Work out the finished part from the listing and answer in its coordinate system (mm). Face numbers are marked on the shaded views. A direction names the side the tool comes from. Give positions to 0.01 mm unless a question says otherwise; leave off trailing zeros. Loops run counter-clockwise (first coordinate to the right, second up) from the corner with the lowest first, then second, coordinate; pieces in that order, holes last. Notation, with made-up numbers: (49.5, 5.5) - (66.5, 5.5) arc R24 cw to (66.5, 28.5) - close; hole circle Ø5 at (-19, -13.75). An arc over 180 degrees is marked (long way). One line per question, with ' | ' between items. Start each with the question number.
1. Which of the six approach directions +Z, -Z, +X, -X, +Y, -Y give full straight-line access (tool end or side, diameter ignored) to the marked faces 1, 2 and 3?
2. Section A-A (y = 28) is taken. Determine the outline of the cut face in (x, z), plus the area to 3 significant figures.
3. Section C-C (y = 83.5) is taken. Determine the outline of the cut face in (x, z), plus the area to 3 significant figures.
4. Each of these flat-tipped pins is pushed along its axis until it touches: pin 1 (0.8 mm diameter, centred on y = 124.5, z = 1.5, fed in from -X); pin 2 (2 mm diameter, centred on y = 72.5, z = 1.5, fed in from +X); pin 3 (8 mm diameter, centred on x = 30, y = 124, fed in from -Z). Where does it stop, or does it pass through?
5. Section D-D (x = -2) is taken. Determine the outline of the cut face in (y, z).
6. Section B-B (x = 10) is taken. Determine the outline of the cut face in (y, z).
7. Find the intervals of material crossed by line 1 (Y direction, x = 10, z = 1); line 2 (X direction, y = 28, z = 0.75); line 3 (X direction, y = 42, z = 1.5), in increasing order.
from build123d import *

# Parameters (mm, degrees)
F1_DEPTH       = 3.5
F3_DEPTH       = 2.5
F5_D           = 4.5
F5_CSINK_D     = 8.96
F5_CSINK_ANGLE = 90


with BuildPart() as f1:
    # F0 (on Top) → F1 (new body)
    with BuildSketch(Plane.XY):
        Polygon((0, 109), (0, 0), (20, 0), (20, 109), (32.5, 124), (32.5, 139), (-12.5, 139), (-12.5, 124), align=None)
    extrude(amount=F1_DEPTH)

    # F2 (on face) → F3 (cut)
    with BuildSketch(Plane(origin=(0, 0, 0), x_dir=(1, 0, 0), z_dir=(0, 0, -1))):
        Polygon((-12.5, -124), (-12.5, -139), (-5, -139), (-5, -115), align=None)
        Polygon((25, -139), (32.5, -139), (32.5, -124), (25, -115), align=None)
    extrude(amount=-F3_DEPTH, mode=Mode.SUBTRACT)

    # F5 (through all)
    with Locations(Plane.XY.offset(3.5)):
        with Locations((10, 98), (10, 28)):
            CounterSinkHole(F5_D / 2, F5_CSINK_D / 2, counter_sink_angle=F5_CSINK_ANGLE)


solid = f1.part
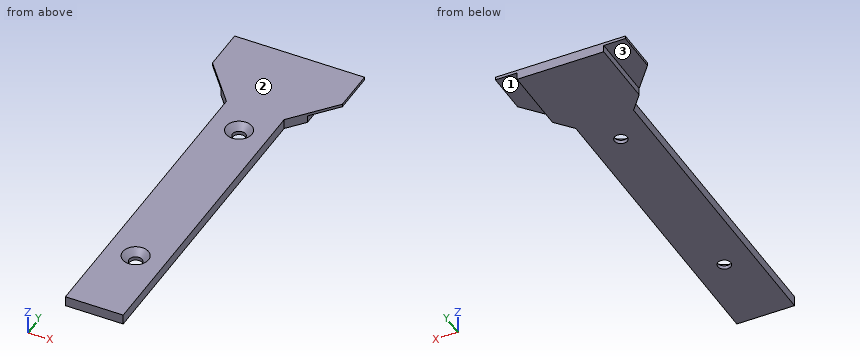
Conclusion:
1) face 1: -Z, +X, +Y, -Y | face 2: +Z, +X, -X, +Y, -Y | face 3: -Z, -X, +Y, -Y
2) outline: (0, 0) - (7.75, 0) - (7.75, 1.27) - (5.52, 3.5) - (0, 3.5) - close; (12.25, 0) - (20, 0) - (20, 3.5) - (14.48, 3.5) - (12.25, 1.27) - close | area: 49.3 mm²
3) outline: (0, 0) - (20, 0) - (20, 3.5) - (0, 3.5) - close | area: 70.0 mm²
4) pin 1: x = -5 | pin 2: x = 20 | pin 3: z = 2.5
5) outline: (111.4, 0) - (139, 0) - (139, 3.5) - (111.4, 3.5) - close
6) outline: (0, 0) - (25.75, 0) - (25.75, 1.27) - (23.52, 3.5) - (0, 3.5) - close; (30.25, 0) - (95.75, 0) - (95.75, 1.27) - (93.52, 3.5) - (32.48, 3.5) - (30.25, 1.27) - close; (100.25, 0) - (139, 0) - (139, 3.5) - (102.48, 3.5) - (100.25, 1.27) - close
7) line 1: 0 to 25.75, 30.25 to 95.75, 100.25 to 139 | line 2: 0 to 7.75, 12.25 to 20 | line 3: 0 to 20
